Geometry: final body of the model. Coordinates: model frame, mm. Face numbers are marked on the shaded views. A direction names the side the tool comes from. Give positions to 0.01 mm unless a question says otherwise; leave off trailing zeros. Write each loop counter-clockwise with the first axis right and the second up, starting at its lowest first coordinate (ties: lowest second). Pieces come first, ordered by that corner, then holes.
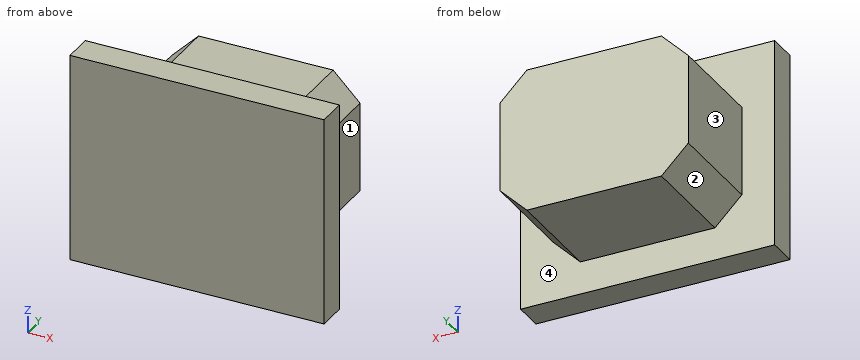
Autodesk Inventor part; units mm, degrees
ref_plane "YZ Plane" through (0, 0, 0) normal (1, 0, 0) x (0, 1, 0)
ref_plane "XZ Plane" through (0, 0, 0) normal (0, 1, 0) x (-1, 0, 0)
ref_plane "XY Plane" through (0, 0, 0) normal (0, 0, 1) x (1, 0, 0)
sketch "Náčrt1" plane through (0, 0, 0) normal (0, 1, 0) x (-1, 0, 0)
  line L0 (0, 0) -> (-8.5, 0)
  line L1 (-8.5, 0) -> (-8.5, -7)
  line L2 (-8.5, -7) -> (0, -7)
  line L3 (0, -7) -> (0, 0)
  dimension "d0" = 8.5
  dimension "d1" = 7
extrude "Vysunutí1" add sketch "Náčrt1" along normal blind 1
sketch "Náčrt2" plane through (0, 1, 0) normal (0, 1, 0) x (1, 0, 0)
  line L0 (1.1, 1.1) -> (7.4, 1.1)
  line L1 (7.4, 1.1) -> (7.4, 5.9)
  line L2 (7.4, 5.9) -> (1.1, 5.9)
  line L3 (1.1, 5.9) -> (1.1, 1.1)
  line L4 (8.5, 7) -> (0, 7)
  line L5 (0, 7) -> (0, 0)
  dimension "d4" = 6.3
  dimension "d5" = 4.8
  dimension "d6" = 1.1
  dimension "d7" = 1.1
extrude "Vysunutí2" add sketch "Náčrt2" along normal blind 3.5
chamfer "Zkosení1" distance 0.9 angle 45 4 edges at (1.1, 2.75, -5.9) (1.1, 2.75, -1.1) (7.4, 2.75, -1.1) (7.4, 2.75, -5.9)
sketch "Náčrt3" plane through (0, 0, 0) normal (0, 0, 1) x (1, 0, 0)
  point P0 (0, 0)
sketch "Náčrt4" plane through (0, 1, 0) normal (0, 1, 0) x (1, 0, 0)
  point P0 (0, 0)
properties part number "MiddleButton"
Q1. Ray query, line 1 along X through (y, z) = (3.85, -4.25); line 2 along Z through (x, y) = (3.5, 3.5); line 3 along Y through (x, z) = (1, -5.5). Return the intervals inside material, ascending.
Filled sheet:
line 1: x = 1.1 to 7.4
line 2: z = -5.9 to -1.1
line 3: y = 0 to 1
Q2. Section D-D on x = 0.75. Output: boundary loops of the cut face in (y, z), plus the area to 3 significant figures.
Filled sheet:
outline: (0, -7) - (1, -7) - (1, 0) - (0, 0) - close
area: 7.00 mm2
Q3. Section A-A on z = -3.25. Output: boundary loops of the cut face in (x, y), plus the area to 4 significant figures.
Filled sheet:
outline: (0, 0) - (8.5, 0) - (8.5, 1) - (7.4, 1) - (7.4, 4.5) - (1.1, 4.5) - (1.1, 1) - (0, 1) - close
area: 30.55 mm2
Q4. Access query for the marked faces 1, 2, 3 and 4. Directions: +Z, -Z, +X, -X, +Y, -Y. A direction counts if a zero-diameter tool reaches every point of the face in a straight line with its end or side. Return the directions, or none.
Filled sheet:
face 1: +Z, -Z, +X, +Y
face 2: -Z, -X, +Y
face 3: +Z, -Z, -X, +Y
face 4: +Y
Q5. Section C-C on z = -6. Output: boundary loops of the cut face in (x, y), plus the area to 3 significant figures.
Filled sheet:
outline: (0, 0) - (8.5, 0) - (8.5, 1) - (0, 1) - close
area: 8.50 mm2
Q6. Section B-B on x = 7. Output: boundary loops of the cut face in (y, z).
Filled sheet:
outline: (0, -7) - (1, -7) - (1, -5.4) - (4.5, -5.4) - (4.5, -1.6) - (1, -1.6) - (1, 0) - (0, 0) - close
Q7. Pin query (flat end, axial travel): P1, Ø0.9, axis at y = 2.5, z = -4, coming from the -X side; P2, Ø2, axis at x = 2.5, y = 1, coming from the +Z side; P3, Ø2, axis at x = 7, y = 3, coming from the +Z side; P4, Ø1, axis at x = 4.5, y = 2.5, coming from the -Z side. Return the tip coordinate at first contact, or that it passes through.
Filled sheet:
P1: stops at x = 1.1
P2: stops at z = 0
P3: stops at z = -1.1
P4: stops at z = -5.9
